CAD build for the part. Positions are in the model's coordinates, mm. A direction names the side the tool comes from. Coordinates: 2 decimals unless noted, no trailing zeros. Order: outer loops, then holes, each group sorted by start corner. A loop starts at its lowest first (then second) coordinate and runs counter-clockwise, first axis right, second up. Notation, with made-up numbers: (51.25, 71) -> (77.25, 71) arc R18 cw to (77.25, 106) -> close; hole circle Ø4 at (-23.5, -27.5). An arc over 180 degrees is marked (long way). Use one line per item in the form item = value. Start each with the question number.
Autodesk Inventor part; units mm, degrees
ref_plane "Work Plane2" through (-23.8125, 0, 0) normal (1, 0, 0) x (0, 1, 0)
ref_plane "XZ Plane" through (0, 0, 0) normal (0, 1, 0) x (-1, 0, 0)
ref_plane "XY Plane" through (0, 0, 0) normal (0, 0, 1) x (1, 0, 0)
sketch "Sketch1" plane through (0, 0, 0) normal (0, 1, 0) x (-1, 0, 0)
  circle A0 centre (0, 0) radius 23.8125
  circle A1 centre (0, 0) radius 63.5
  dimension "d2" = 127
  dimension "d8" = 47.625
extrude "Extrusion1" add sketch "Sketch1" along normal blind 1314.45 contours A0
extrude "Extrusion2" add sketch "Sketch1" along normal blind 19.05
sketch "Sketch3" plane through (0, 1314.45, 0) normal (0, 1, 0) x (1, 0, 0)
  circle A0 centre (0, 0) radius 23.8125
  circle A1 centre (0, 0) radius 63.5
  dimension "d5" = 127
extrude "Extrusion3" add sketch "Sketch3" against normal blind 19.05
sketch "Sketch4" plane through (0, 1314.45, 0) normal (0, 1, 0) x (1, 0, 0)
  circle A0 centre (0, 0) radius 63.5
  line L0 (0, 63.5) -> (0, -63.5)
  line L1 (63.5, 0) -> (-63.5, 0)
  circle A1 centre (44.45, 31.3787) radius 7.9375
  circle A2 centre (0, 0) radius 19.05
  circle A3 centre (44.45, -31.3787) radius 7.9375
  circle A4 centre (-44.45, 31.3787) radius 7.9375
  circle A5 centre (-44.45, -31.3787) radius 7.9375
  line L2 (0, 0) -> (-44.9013, 44.9013)
  line L3 (0, 0) -> (44.9013, 44.9013)
  point P0 (-22.4506, 22.4506)
  dimension "d9" = 38.1
  dimension "d12" = 44.45
  dimension "d13" = 15.875
  dimension "d26" = 45
  dimension "d28" = 45
extrude "Extrusion4" cut sketch "Sketch4" against normal blind 1314.45 contours A2 L0 L1 | L1 L3 A2 | L3 L0 A2 | A2 L1 L0 | L2 A2 L0 | L1 A2 L2
extrude "Extrusion5" cut sketch "Sketch4" against normal blind 1314.45 contours A1 | A3 | A4 | A5
ref_plane "Work Plane1" through (-63.5, 0, 0) normal (1, 0, 0) x (0, 1, 0)
sketch "Sketch5" plane through (-63.5, 0, 0) normal (1, 0, 0) x (0, 1, 0)
  line L0 (1314.45, 19.05) -> (0, 19.05)
  line L1 (1111.25, 19.05) -> (1111.25, -14.2371)
  line L2 (1314.45, -63.5) -> (1314.45, 63.5)
  circle A0 centre (1111.25, 0) radius 6.35
  point P0 (0, 0)
  dimension "d17" = 203.2
  dimension "d18" = 12.7
extrude "Extrusion6" cut sketch "Sketch5" along normal blind 44.45
thread "Thread1"
ref_plane "Work Plane2" through (-23.8125, 0, 0) normal (1, 0, 0) x (0, 1, 0)
sketch "Sketch6" plane through (-63.5, 0, 0) normal (1, 0, 0) x (0, 1, 0)
  line L0 (4.6815, -69.7945) -> (23.2887, -69.7945)
  line L1 (23.2887, -69.7945) -> (1344.0887, -69.7945)
  line L2 (683.6887, -69.7945) -> (683.6887, -90.3747)
  line L3 (683.6887, -69.7945) -> (683.6887, -37.5296)
  line L4 (683.6887, -69.7945) -> (715.9537, -69.7945) construction
  point P0 (0, 0)
  dimension "d23" = 1320.8
  dimension "d24" = 90
ref_plane "Work Plane3" through (0, 1314.45, 0) normal (0.7071, 0, -0.7071) x (-0.7071, 0, -0.7071)
ref_plane "Work Plane4" through (0, 1314.45, 0) normal (-0.7071, 0, -0.7071) x (0.7071, 0, -0.7071)
properties part number "New Metal Pipe"
1) Probe L1, parallel to X at y = 737.5, z = 0.5; L2, parallel to Y at x = -20.4, z = 0; L3, parallel to Y at x = 26, z = -57. List the from-to ranges inside material, lowest first.
2) Drop flat-ended pins along their axis: P1, Ø1.5, axis at x = -20.5, y = 1025.5, coming from the +Z side; P2, Ø8, axis at x = -31.5, z = 1, coming from the -Y side; P3, Ø1.5, axis at x = -17, y = 1156.5, coming from the +Z side; P4, Ø4, axis at x = -15.5, y = 1067.5, coming from the -Z side. Give the stop position or say it passes through.
3) 3-axis set-ups, long thin cutter, end or side, ignore diameter. For faces 1 (the face through (27, 1295.4, -1)), 2 (the face through (-13, 0, 15)): which of +Z, -Z, +X, -X, +Y, -Y reach the whole face in a straight line?
4) Two-plate mould, pull along Y, no slides. Class faces 3 (the face through (-27, 19.05, 1)), 4 (the face through (13, 1314.45, -15)), 5 (the face through (-15.12, 666.43, 11.59)): released by +Y, released by -Y, zero draft, split by the parting line, or undercut.
5) Cut at A-A on x = 0. Give the cut face in (y, z), then the cut area to 3 significant figures.
Values follow:
q1.L1 = -23.81 to -19.04, 19.04 to 23.81
q1.L2 = 0 to 1104.9, 1117.6 to 1314.45
q1.L3 = 0 to 19.05, 1295.4 to 1314.45
q2.P1 = 13.3
q2.P2 = 0
q2.P3 = 17.41
q2.P4 = -19.62
q3.face_1 = none
q3.face_2 = +Z, -Z, +X, -X, -Y
q4.face_3 = undercut
q4.face_4 = released by +Y
q4.face_5 = zero draft
q5.outline = (0, -63.5) -> (19.05, -63.5) -> (19.05, -23.81) -> (1295.4, -23.81) -> (1295.4, -63.5) -> (1314.45, -63.5) -> (1314.45, -19.05) -> (0, -19.05) -> close; (0, 19.05) -> (1314.45, 19.05) -> (1314.45, 63.5) -> (1295.4, 63.5) -> (1295.4, 23.81) -> (19.05, 23.81) -> (19.05, 63.5) -> (0, 63.5) -> close
q5.area = 15,500 mm^2
